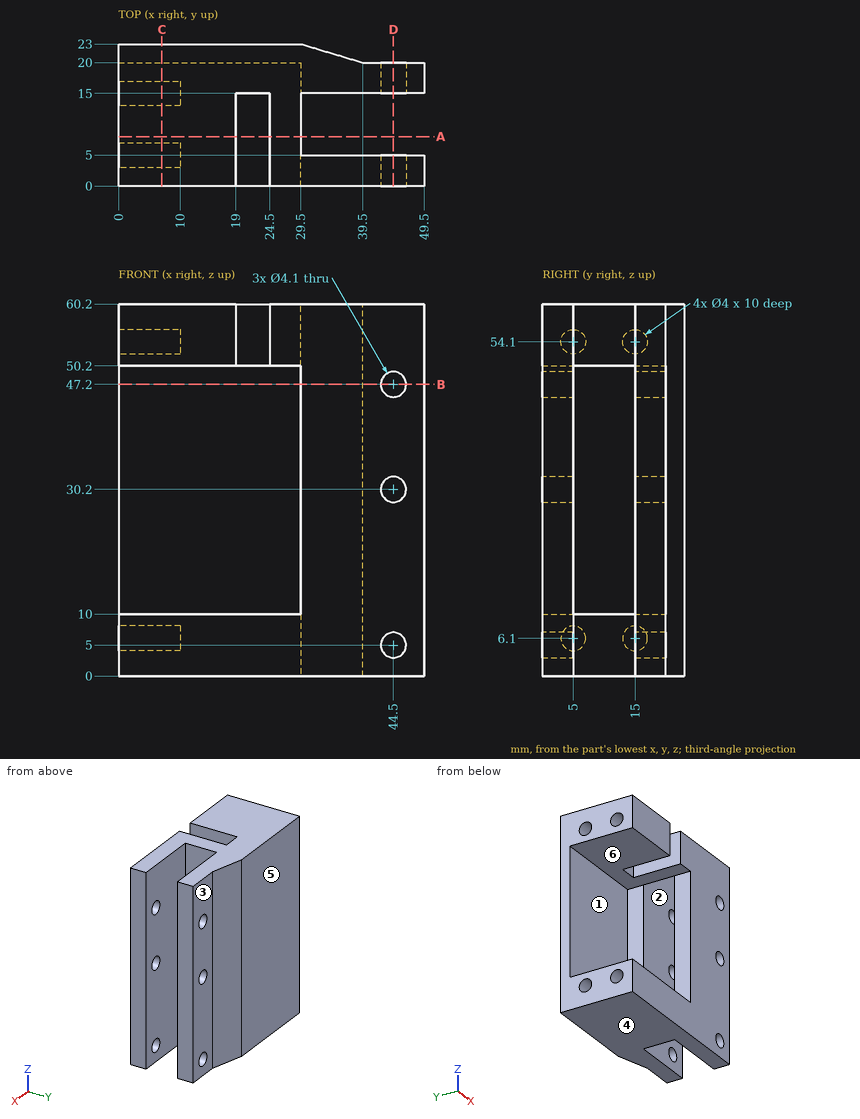
Input: dimensioned drawing with shaded views. Units: mm. Origin: part minimum x, y, z. A direction names the side the tool comes from. Coordinates: 2 decimals unless noted, no trailing zeros. Write each loop counter-clockwise with the first axis right and the second up, starting at its lowest first coordinate (ties: lowest second). Pieces come first, ordered by that corner, then holes. Notation, with made-up numbers: (12.25, 48.25) -> (53.25, 48.25) arc R21 ccw to (53.25, 87.25) -> close; hole circle Ø10 at (27, -2). An arc over 180 degrees is marked (long way). Return JSON: item names as keys, results as strings. Group by question number.
1) Set-up query: the marked faces 1, 2 and 3. Return all of +Z, -Z, +X, -X, +Y, -Y with unobstructed straight access to the full face (end or side cutting, diameter ignored); none if empty.
2) Section query C-C, the plane x = 7. Return loops of the section in (y, z), plus the area to 3 significant figures.
3) Ray query, line 1 along X through (y, z) = (1.8, 47.2); line 2 along Y through (x, z) = (44, 8.5); line 3 along Z through (x, y) = (10, 9). Return the intervals inside material, ascending.
4) Section query B-B, the plane z = 47.2. Return loops of the section in (x, y).
5) Section query D-D, the plane x = 44.5. State how many separate pieces and enclosed holes the cut face has, plus the area to 3 significant figures.
6) Contact query for flat-ended pins moving along their axis: P1, Ø5.5, axis at y = 3, z = 23, coming from the -X side; P2, Ø10, axis at x = 44, z = 38.5, coming from the +Y side; P3, Ø5.5, axis at x = 44.5, z = 30.2, coming from the +Y side. Output: stop coordinate, or through.
7) Section query A-A, the plane y = 8. Return loops of the section in (x, z).
8) Mould query, pull axis Z, two halves, no side actions, for the marked faces 4, 5 and 6. Classes: +Z half, -Z half, draft (parallel to the pull), parting line (faces both ways), or undercut.
From the geometry:
{
 "1": {"face 1": "-X, -Y", "face 2": "+Z, -Z, +X", "face 3": "+Z, -Z, +X, +Y"},
 "2": {"outline": "(0, 0) -> (23, 0) -> (23, 60.2) -> (0, 60.2) -> (0, 50.2) -> (20, 50.2) -> (20, 10) -> (0, 10) -> close; hole circle Ø4 at (5, 6.1); hole circle Ø4 at (5, 54.1); hole circle Ø4 at (15, 6.1); hole circle Ø4 at (15, 54.1)", "area": "530 mm²"},
 "3": {"line 1": "29.5 to 42.45, 46.55 to 49.5", "line 2": "0 to 5, 15 to 20", "line 3": "0 to 10, 50.2 to 60.2"},
 "4": {"outline": "(0, 20) -> (29.5, 20) -> (29.5, 15) -> (42.45, 15) -> (42.45, 20) -> (39.5, 20) -> (29.5, 23) -> (0, 23) -> close; (29.5, 0) -> (42.45, 0) -> (42.45, 5) -> (29.5, 5) -> close; (46.55, 0) -> (49.5, 0) -> (49.5, 5) -> (46.55, 5) -> close; (46.55, 15) -> (49.5, 15) -> (49.5, 20) -> (46.55, 20) -> close"},
 "5": {"separate pieces": "8", "enclosed holes": "0", "area": "479 mm²"},
 "6": {"P1": "x = 29.5", "P2": "y = 20.15", "P3": "y = 20"},
 "7": {"outline": "(0, 0) -> (29.5, 0) -> (29.5, 10) -> (0, 10) -> close; (0, 50.2) -> (19, 50.2) -> (19, 60.2) -> (0, 60.2) -> close; (24.5, 50.2) -> (29.5, 50.2) -> (29.5, 60.2) -> (24.5, 60.2) -> close"},
 "8": {"face 4": "-Z half", "face 5": "draft", "face 6": "undercut"}
}
